Print and shaded views of the part. All mm, measured from the part's lowest x, y and z. Give positions to 0.01 mm unless a question says otherwise; leave off trailing zeros. Loops run counter-clockwise (first coordinate to the right, second up) from the corner with the lowest first, then second, coordinate; pieces in that order, holes last. Notation, with made-up numbers: (5.25, 5) - (11.25, 5) arc R19 cw to (11.25, 29) - close; hole circle Ø4 at (33.25, -30.75). An arc over 180 degrees is marked (long way). Return JSON: item names as keys, results as strings.
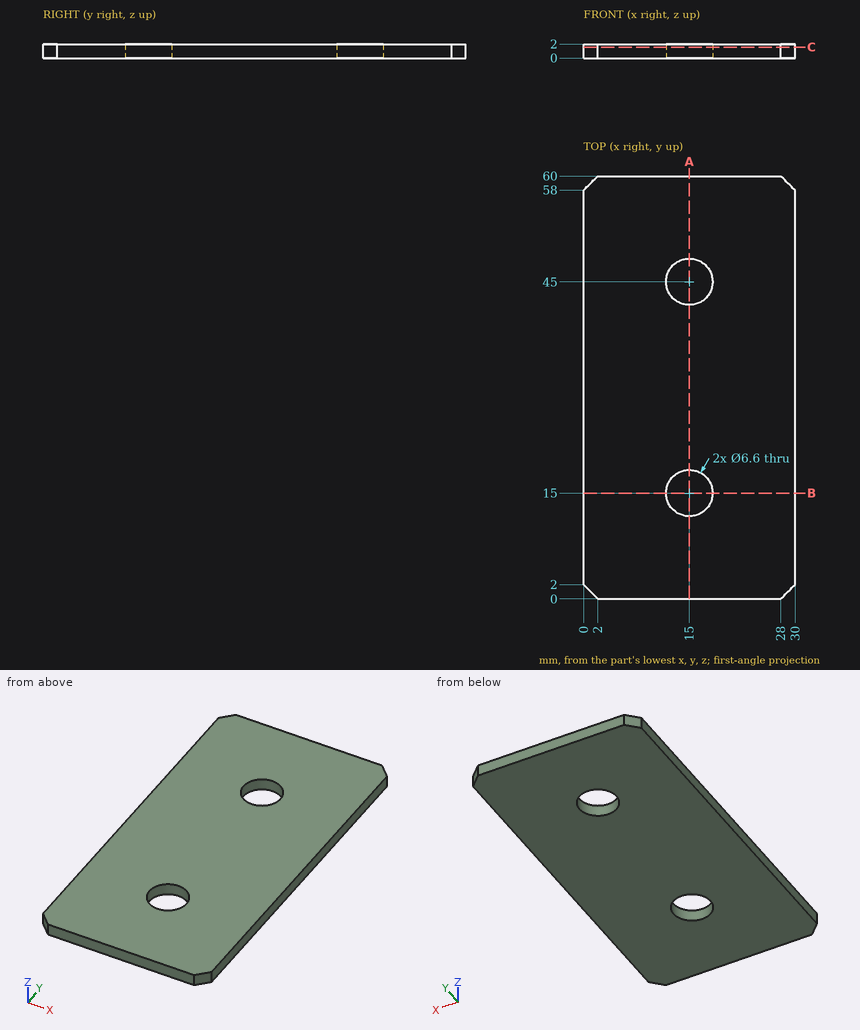
1. Cut at C-C, the plane z = 1.55. Write the cut outline in (x, y).
Values follow:
{"outline": "(0, 2) - (2, 0) - (28, 0) - (30, 2) - (30, 58) - (28, 60) - (2, 60) - (0, 58) - close; hole circle Ø6.6 at (15, 15); hole circle Ø6.6 at (15, 45)"}
2. Drill centre lines: probe 1 along Y at (x, z) = (15, 0.4); probe 2 along Y at (x, z) = (13.25, 0.4); probe 3 along X at (y, z) = (46, 1.9). Where is each one in solid material? Low to high.
Values follow:
{"probe 1": "y = 0 to 11.7, 18.3 to 41.7, 48.3 to 60", "probe 2": "y = 0 to 12.2, 17.8 to 42.2, 47.8 to 60", "probe 3": "x = 0 to 11.86, 18.14 to 30"}
3. Cut at B-B, the plane y = 15. Write the cut outline in (x, z).
Values follow:
{"outline": "(0, 0) - (11.7, 0) - (11.7, 2) - (0, 2) - close; (18.3, 0) - (30, 0) - (30, 2) - (18.3, 2) - close"}
4. Cut at A-A, the plane x = 15. Write the cut outline in (y, z).
Values follow:
{"outline": "(0, 0) - (11.7, 0) - (11.7, 2) - (0, 2) - close; (18.3, 0) - (41.7, 0) - (41.7, 2) - (18.3, 2) - close; (48.3, 0) - (60, 0) - (60, 2) - (48.3, 2) - close"}
